from build123d import *

# Parameters (mm, degrees)
SKETCH_2_W          = 15.8
SKETCH_2_H          = 15.8
EXTRUDE_1_DEPTH     = 9.6
SKETCH_3_W          = 8
SKETCH_3_H          = 8
CUT_EXTRUDE_1_DEPTH = 9.6
SKETCH_4_R          = 2.4
EXTRUDE_2_DEPTH     = 1.7
SKETCH_5_R          = 2.5
CUT_EXTRUDE_2_DEPTH = 1.8


with BuildPart() as part:
    # Эскиз2 → Бобышка-Вытянуть1 (new body)
    with BuildSketch(Plane(origin=(0, 0, 0), x_dir=(1, 0, 0), z_dir=(0, 1, 0))):
        Rectangle(SKETCH_2_W, SKETCH_2_H)
    extrude(amount=EXTRUDE_1_DEPTH)

    # Эскиз3 → Вырез-Вытянуть1 (cut)
    with BuildSketch(Plane(origin=(0, 9.6, 0), x_dir=(1, 0, 0), z_dir=(0, 1, 0))):
        with Locations((-3.9, -3.9)):
            Rectangle(SKETCH_3_W, SKETCH_3_H)
    extrude(amount=-CUT_EXTRUDE_1_DEPTH, mode=Mode.SUBTRACT)

    # Эскиз4 → Бобышка-Вытянуть2 (add)
    with BuildSketch(Plane(origin=(0, 9.6, 0), x_dir=(1, 0, 0), z_dir=(0, 1, 0))):
        with Locations(Location((-4, 4, 0), (0, 0, 270))):
            Circle(SKETCH_4_R)
        with Locations(Location((4, 4, 0), (0, 0, 270))):
            Circle(SKETCH_4_R)
        with Locations(Location((4, -4, 0), (0, 0, 270))):
            Circle(SKETCH_4_R)
    extrude(amount=EXTRUDE_2_DEPTH)

    # Эскиз5 → Вырез-Вытянуть2 (cut)
    with BuildSketch(Plane.XZ):
        with Locations(Location((-4, -4, 0), (0, 0, 270))):
            Circle(SKETCH_5_R)
        with Locations(Location((4, -4, 0), (0, 0, 270))):
            Circle(SKETCH_5_R)
        with Locations(Location((4, 4, 0), (0, 0, 270))):
            Circle(SKETCH_5_R)
    extrude(amount=-CUT_EXTRUDE_2_DEPTH, mode=Mode.SUBTRACT)


solid = part.part
Work out the finished part from the listing and answer in its coordinate system (mm). A direction names the side the tool comes from. Round coordinates to 2 decimals unless told otherwise and drop trailing zeros. Loops run counter-clockwise (first coordinate to the right, second up) from the corner with the lowest first, then second, coordinate; pieces in that order, holes last. Notation, with made-up numbers: M 37.5,18 L 63.5,18 A36 cw 63.5,54 Z; hole C -32.5,85 d9. An arc over 180 degrees is marked long. One line per question, with ' | ' between items. Start each with the question number.
(1) A cutting plane is placed at B-B on z = 4. Write down the section's boundary in (x, y).
(2) A cutting plane is placed at D-D on y = 7.5. Write down the section's boundary in (x, z), plus the area to 3 significant figures.
(3) For a pull along X with two mould halves and no side action, classify faces 5 (the face through (6.024, 10.438, 5.29)), 6 (the face through (4, 11.3, -4)), 7 (the face through (4.751, 0.887, 1.615)) as released by +X, released by -X, zero draft, split by the parting line, or undercut.
(4) A cutting plane is placed at A-A on y = 1.5. Write down the section's boundary in (x, z).
(5) Flat-ended cylindrical pins translate along their axes: pin 1 Ø6.5 at (x, y) = (-5, 3.5) entering from +Z; pin 2 Ø6.5 at (y, z) = (2.5, 6) entering from -X; pin 3 Ø4.5 at (x, z) = (-0.5, 2.5) entering from +Y. Find the tip coordinate at first contact, or state that the pin passes through.
(6) A tool of negligible diameter and unlimited length cuts with its end or side. For faces 1 (the face through (6.024, 10.438, -2.71)), 2 (the face through (-3.249, 0.887, -6.385)), 3 (the face through (0.1, 5, 4)), 4 (the face through (7.9, 5, 0)), from which of +Z, -Z, +X, -X, +Y, -Y can it reach the whole face along a straight path? Write none if from no direction.
(7) Find the intervals of material crossed by line 1 (X direction, y = 1.2, z = -4); line 2 (X direction, y = 1.05, z = 4); line 3 (X direction, y = 5, z = 7), in increasing order.
(8) A cutting plane is placed at C-C on x = 4. Write down the section's boundary in (y, z).
Geometry check:
1) outline: M 0.1,0 L 1.5,0 L 1.5,1.8 L 6.5,1.8 L 6.5,0 L 7.9,0 L 7.9,9.6 L 6.4,9.6 L 6.4,11.3 L 1.6,11.3 L 1.6,9.6 L 0.1,9.6 Z
2) outline: M -7.9,-7.9 L 7.9,-7.9 L 7.9,7.9 L 0.1,7.9 L 0.1,-0.1 L -7.9,-0.1 Z | area: 186 mm²
3) face 5: split by the parting line | face 6: zero draft | face 7: undercut
4) outline: M -7.9,-7.9 L 7.9,-7.9 L 7.9,7.9 L 0.1,7.9 L 0.1,-0.1 L -7.9,-0.1 Z; hole C -4,-4 d5; hole C 4,-4 d5; hole C 4,4 d5
5) pin 1: stops at z = -0.1 | pin 2: stops at x = 0.1 | pin 3: stops at y = 9.6
6) face 1: +Y | face 2: -Y | face 3: +Z, -X, +Y, -Y | face 4: +Z, -Z, +X, +Y, -Y
7) line 1: x = -7.9 to -6.5, -1.5 to 1.5, 6.5 to 7.9 | line 2: x = 0.1 to 1.5, 6.5 to 7.9 | line 3: x = 0.1 to 7.9
8) outline: M 0,-7.9 L 9.6,-7.9 L 9.6,-6.4 L 11.3,-6.4 L 11.3,-1.6 L 9.6,-1.6 L 9.6,1.6 L 11.3,1.6 L 11.3,6.4 L 9.6,6.4 L 9.6,7.9 L 0,7.9 L 0,6.5 L 1.8,6.5 L 1.8,1.5 L 0,1.5 L 0,-1.5 L 1.8,-1.5 L 1.8,-6.5 L 0,-6.5 Z
